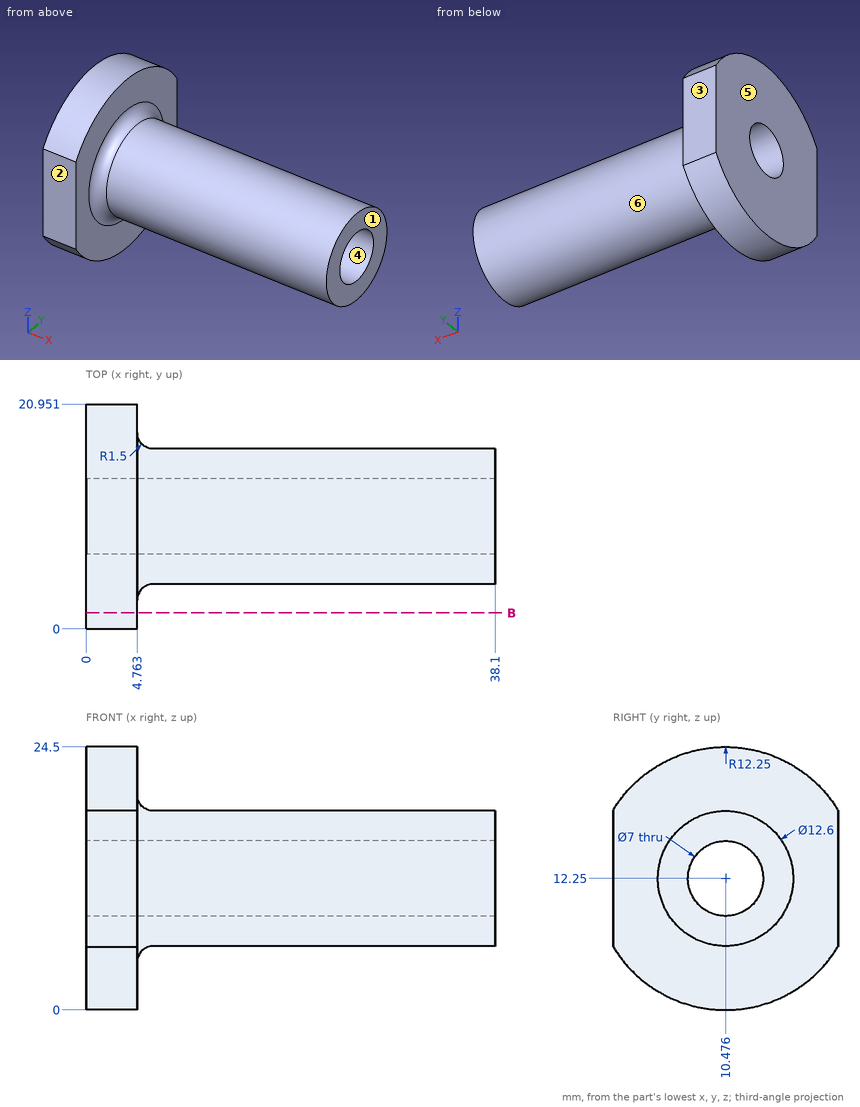
Answer from the drawing. Dimensions are ordinates in mm from the lowest x, y and z of the part. A direction names the side the tool comes from. Coordinates: 2 decimals unless noted, no trailing zeros. Write each loop counter-clockwise with the first axis right and the second up, starting at its lowest first coordinate (ties: lowest second). Pieces come first, ordered by that corner, then holes. Notation, with made-up numbers: M -17.5,-13.5 L 39.5,-13.5 A35 ccw 39.5,22.5 Z; hole C -36.5,-30 d10. An arc over 180 degrees is marked long. Use one line per item in the form item = value. Start each with the question number.
1. The part is cut by section B-B (y = 1.5). Give the vertices of the cut face in (x, z), plus the area to 3 significant figures.
2. The mould has two halves that part along Y. Classify the marked faces 1, 2, 3 and 4: released by +Y, released by -Y, zero draft, split by the parting line, or undercut.
3. Each of these flat-tipped pins is pushed along its axis until it touches: P1, Ø3, axis at x = 13.5, z = 17, coming from the +Y side; P2, Ø6, axis at x = 33, y = 18.5, coming from the -Z side. Where does it stop, or does it pass through?
4. Straight lines are drawn through the part: probe 1 along Y at (x, z) = (12.5, 12.25) (1 decimal); probe 2 along X at (y, z) = (14, 19.5); probe 3 along Z at (x, y) = (15.5, 10). For each, find the intervals that lie inside material, in ascending order. Write a range as from..to.
5. A tool of negligible diameter and unlimited length cuts with its end or side. For the marked faces 5 and 6, from which of +Z, -Z, +X, -X, +Y, -Y can it reach the whole face along a straight path? Write none if from no direction.
Evaluation:
q1.outline = M 0,3.91 L 4.76,3.91 L 4.76,20.59 L 0,20.59 Z
q1.area = 79.4 mm^2
q2.face_1 = zero draft
q2.face_2 = released by -Y
q2.face_3 = released by +Y
q2.face_4 = undercut
q3.P1 = 15.87
q3.P2 = 8.45
q4.probe_1 = 4.2..7, 14..16.8
q4.probe_2 = 0..4.76
q4.probe_3 = 5.97..8.78, 15.72..18.53
q5.face_5 = +Z, -Z, -X, +Y, -Y
q5.face_6 = +X
